Model file for the job. Use its own axes, mm. A direction names the side the tool comes from. Coordinates: 2 decimals unless noted, no trailing zeros. Write each loop counter-clockwise with the first axis right and the second up, starting at its lowest first coordinate (ties: lowest second). Pieces come first, ordered by that corner, then holes.
Q1. Band-saw the part on C-C, the plane x = -61.5. Write the cut outline in (y, z).
Q2. Drill centre lines: probe 1 along X at (y, z) = (3.5, 2) (3 decimals); probe 2 along X at (y, z) = (7, 11); probe 3 along X at (y, z) = (5.75, 2). Where is each one in solid material? Low to high.
Q3. Band-saw the part on B-B, the plane x = 25. Write the cut outline in (y, z).
Q4. Pin check, flat tips, straight feed: P1, Ø1.5, axis at x = -43.5, z = 4.5, coming from the -Y side; P2, Ø6, axis at x = -3, z = 8.5, coming from the +Y side; P3, Ø3.5, axis at x = -45.5, z = 7, coming from the +Y side; P4, Ø1, axis at x = -60.5, z = 2, coming from the -Y side. Stop position of each tip, or through.
Q5. Which spindle directions (+Z, -Z, +X, -X, +Y, -Y) get a long thin tool onto all of the face, cutting with end or side? Do faces 3 (the flat face through (76.66, 3.77, 4.34)), 4 (the cylindrical face through (60.16, 11.75, 5.92)), 5 (the flat face through (-64, 2, 6)). Say none if no direction does.
Q6. Pull direction Z, two halves, no side cores. Call faces 1 (the flat face through (64, 2, 6)), 2 (the flat face through (-49.015, 3.768, 7.615)): released by +Z, released by -Z, zero draft, split by the parting line, or undercut.
Q7. Band-saw the part on A-A, the plane y = 9.75. Write the cut outline in (x, z), plus the area to 3 significant figures.
from build123d import *

# Parameters (mm, degrees)
F0_W     = 3.875
F0_H     = 3.875
F1_DEPTH = 12
F3_DEPTH = 2.5
F4_R     = 1.5
F5_DEPTH = 5.001


# Not quite as in the source:
# - a pattern or mirror of a feature is missing from the dataset's text; its kind, count and spacing are read off the source's solid
# - a feature names something its author has since deleted; it is built from what else it names


with BuildPart() as f1:
    # F0 (on Top) → F1 (new body)
    with BuildSketch(Plane.XY):
        with BuildLine():
            Line((-67.7942286341, 5), (-79.875, 5))
            Line((-79.875, 5), (-79.875, 0))
            Line((-79.875, 0), (-67.875, 0))
            Line((-67.875, 0), (-67.875, 3.875))
            ThreePointArc((-67.875, 3.875), (-67.854781203, 4.4389479173), (-67.7942286341, 5))
        make_face()
        with BuildLine():
            ThreePointArc((-52.2057713659, 5), (-60, 11.75), (-67.7942286341, 5))
            Line((-67.7942286341, 5), (-63.8385381332, 5))
            ThreePointArc((-63.8385381332, 5), (-60, 7.875), (-56.1614618668, 5))
            Line((-56.1614618668, 5), (-52.2057713659, 5))
        make_face()
        with BuildLine():
            Line((-63.8385381332, 5), (-67.7942286341, 5))
            ThreePointArc((-67.7942286341, 5), (-67.854781203, 4.4389479173), (-67.875, 3.875))
            Line((-67.875, 3.875), (-64, 3.875))
            ThreePointArc((-64, 3.875), (-63.9594287803, 4.4432637888), (-63.8385381332, 5))
        make_face()
        with BuildLine():
            ThreePointArc((-52.125, 3.875), (-52.145218797, 4.4389479173), (-52.2057713659, 5))
            Line((-52.2057713659, 5), (-56.1614618668, 5))
            ThreePointArc((-56.1614618668, 5), (-56.0405712197, 4.4432637888), (-56, 3.875))
            Line((-56, 3.875), (-52.125, 3.875))
        make_face()
        with BuildLine():
            Line((52.2057713659, 5), (-52.2057713659, 5))
            ThreePointArc((-52.2057713659, 5), (-52.145218797, 4.4389479173), (-52.125, 3.875))
            Line((-52.125, 3.875), (-52.125, 0))
            Line((-52.125, 0), (52.125, 0))
            Line((52.125, 0), (52.125, 3.875))
            ThreePointArc((52.125, 3.875), (52.145218797, 4.4389479173), (52.2057713659, 5))
        make_face()
        with Locations((-65.9375, 1.9375)):
            Rectangle(F0_W, F0_H)
        with BuildLine():
            ThreePointArc((67.7942286341, 5), (60, 11.75), (52.2057713659, 5))
            Line((52.2057713659, 5), (56.1614618668, 5))
            ThreePointArc((56.1614618668, 5), (60, 7.875), (63.8385381332, 5))
            Line((63.8385381332, 5), (67.7942286341, 5))
        make_face()
        with BuildLine():
            Line((56.1614618668, 5), (52.2057713659, 5))
            ThreePointArc((52.2057713659, 5), (52.145218797, 4.4389479173), (52.125, 3.875))
            Line((52.125, 3.875), (56, 3.875))
            ThreePointArc((56, 3.875), (56.0405712197, 4.4432637888), (56.1614618668, 5))
        make_face()
        with Locations((-54.0625, 1.9375)):
            Rectangle(F0_W, F0_H)
        with BuildLine():
            ThreePointArc((67.875, 3.875), (67.854781203, 4.4389479173), (67.7942286341, 5))
            Line((67.7942286341, 5), (63.8385381332, 5))
            ThreePointArc((63.8385381332, 5), (63.9594287803, 4.4432637888), (64, 3.875))
            Line((64, 3.875), (67.875, 3.875))
        make_face()
        with BuildLine():
            Line((79.875, 5), (67.7942286341, 5))
            ThreePointArc((67.7942286341, 5), (67.854781203, 4.4389479173), (67.875, 3.875))
            Line((67.875, 3.875), (67.875, 0))
            Line((67.875, 0), (79.875, 0))
            Line((79.875, 0), (79.875, 5))
        make_face()
        with Locations((54.0625, 1.9375)):
            Rectangle(F0_W, F0_H)
        with Locations((65.9375, 1.9375)):
            Rectangle(F0_W, F0_H)
    extrude(amount=F1_DEPTH)

    # F2 (on face) → F3 (cut)
    with BuildSketch(Plane(origin=(0, 5, 0), x_dir=(-1, 0, 0), z_dir=(0, 1, 0))):
        Polygon((44.2745635514, 2.725), (48.0562078146, 2.725), (49.9470299462, 6), (48.0562078146, 9.275), (44.2745635514, 9.275), (42.3837414198, 6), align=None)
        Polygon((71.9437921854, 2.725), (75.7254364486, 2.725), (77.6162585802, 6), (75.7254364486, 9.275), (71.9437921854, 9.275), (70.0529700538, 6), align=None)
    f3 = extrude(amount=-F3_DEPTH, mode=Mode.SUBTRACT)

    # F3_copies: F3 across plane
    add(f3.mirror(Plane(origin=(0, 0, 0), x_dir=(0, 0, 1), z_dir=(1, 0, 0))), mode=Mode.SUBTRACT)

    # F4 (on face) → F5 (cut, through all)
    with BuildSketch(Plane(origin=(0, 5, 0), x_dir=(-1, 0, 0), z_dir=(0, 1, 0))):
        with Locations((46.165385683, 6)):
            Circle(F4_R)
        with Locations((73.834614317, 6)):
            Circle(F4_R)
    f5 = extrude(amount=-F5_DEPTH, mode=Mode.SUBTRACT)

    # F5_copies: F5 across plane
    add(f5.mirror(Plane(origin=(0, 0, 0), x_dir=(0, 0, 1), z_dir=(1, 0, 0))), mode=Mode.SUBTRACT)


solid = f1.part
Answer sheet:
1. outline: (7.58, 0) - (11.61, 0) - (11.61, 12) - (7.58, 12) - close
2. probe 1: x = -79.875 to -64, -56 to 56, 64 to 79.875
2. probe 2: x = -67.23 to -62.5, -57.5 to -52.77, 52.77 to 57.5, 62.5 to 67.23
2. probe 3: x = -67.65 to -63.53, -56.47 to -52.35, 52.35 to 56.47, 63.53 to 67.65
3. outline: (0, 0) - (5, 0) - (5, 12) - (0, 12) - close
4. P1: stops at y = 0
4. P2: stops at y = 5
4. P3: stops at y = 2.5
4. P4: stops at y = 7.75
5. face 3: +Y
5. face 4: +Z, -Z, +Y
5. face 5: +Z, -Z, -Y
6. face 1: zero draft
6. face 2: undercut
7. outline: (-65.24, 0) - (-54.76, 0) - (-54.76, 12) - (-65.24, 12) - close; (54.76, 0) - (65.24, 0) - (65.24, 12) - (54.76, 12) - close
7. area: 252 mm2
